Autodesk Fusion 360 part; units mm, degrees
sketch "Sketch1" plane through (0, 0, 0) normal (0, 1, 0) x (1, 0, 0)
  line L0 (-25, 0) -> (15, 0)
  line L1 (15, 0) -> (15, -10)
  line L2 (15, -10) -> (-25, -10)
  line L3 (-25, -10) -> (-25, 0)
  dimension "d1" = 40
  dimension "d2" = 10
extrude "Extrude1" add sketch "Sketch1" along normal blind 16
sketch "Sketch2" plane through (0, 16, 0) normal (0, 1, 0) x (-1, 0, 0)
  line L0 (25, 10) -> (-15, 10)
  line L1 (-15, 10) -> (-15, 0)
  line L2 (-15, 0) -> (25, 0)
  line L3 (25, 0) -> (25, 10)
  line L4 (-15, 10) -> (-3, 10)
  line L5 (-3, 10) -> (-3, 9)
  line L6 (-3, 9) -> (6.5, 9)
  line L7 (6.5, 9) -> (6.5, 1)
  line L8 (6.5, 1) -> (-3, 1)
  line L9 (-3, 1) -> (-3, 9)
  dimension "d5" = 12
  dimension "d6" = 9.5
  dimension "d7" = 8
extrude "Extrude2" cut sketch "Sketch2" against normal blind 50 contours L6 L7 L8 L9
sketch "Sketch3" plane through (0, 0, 10) normal (0, 0, 1) x (1, 0, 0)
  line L0 (-25, 0) -> (15, 0)
  line L1 (15, 0) -> (15, 16)
  line L2 (15, 16) -> (-25, 16)
  line L3 (-25, 16) -> (-25, 0)
  line L4 (15, 16) -> (3, 16)
  line L5 (3, 16) -> (3, 12.75)
  line L6 (3, 12.75) -> (-6.5, 12.75)
  line L7 (-6.5, 12.75) -> (-6.5, 16)
  line L8 (-6.5, 16) -> (3, 16)
  line L9 (3, 16) -> (3, 12.75)
  line L10 (-6.5, 12.75) -> (3, 12.75)
  line L11 (3, 12.75) -> (3, -1)
  line L12 (3, -1) -> (-6.5, -1)
  line L13 (-6.5, -1) -> (-6.5, 12.75)
  dimension "d10" = 12
  dimension "d11" = 3.25
  dimension "d12" = 9.5
extrude "Extrude3" cut sketch "Sketch3" against normal blind 50 contours L0 L6 L10 L11 L13
sketch "Sketch4" plane through (0, 0, 10) normal (0, 0, 1) x (1, 0, 0)
  line L0 (-6.5, 0) -> (-6.5, 12.75)
  line L1 (-6.5, 12.75) -> (3, 12.75)
  line L2 (3, 12.75) -> (3, 0)
  line L3 (3, 0) -> (15, 0)
  line L4 (15, 0) -> (15, 16)
  line L5 (15, 16) -> (-25, 16)
  line L6 (-25, 16) -> (-25, 0)
  line L7 (-25, 0) -> (-6.5, 0)
  line L8 (-25, 12.75) -> (-20, 12.75)
  line L9 (-20, 12.75) -> (-20, -3.5611)
  line L10 (-20, -3.5611) -> (-25, -3.5611)
  line L11 (-25, -3.5611) -> (-25, 12.75)
  line L12 (15, 12.75) -> (10, 12.75)
  line L13 (10, 12.75) -> (10, -3.5611)
  line L14 (10, -3.5611) -> (15, -3.5611)
  line L15 (15, -3.5611) -> (15, 12.75)
  dimension "d15" = 5
  dimension "d16" = 5
extrude "Extrude4" cut sketch "Sketch4" against normal blind 50 contours L7 L9 L10 L11 | L6 L7 L8 L9 L11 | L3 L4 L12 L13 L15 | L3 L13 L14 L15
sketch "Sketch5" plane through (0, 16, 0) normal (0, 1, 0) x (-1, 0, 0)
  line L0 (6.5, 9) -> (6.5, 1)
  line L1 (6.5, 1) -> (-3, 1)
  line L2 (-3, 1) -> (-3, 9)
  line L3 (-3, 9) -> (6.5, 9)
  line L4 (25, 10) -> (-15, 10)
  line L5 (-15, 10) -> (-15, 0)
  line L6 (-15, 0) -> (25, 0)
  line L7 (25, 0) -> (25, 10)
  line L8 (-3, 1) -> (-5.5, 1)
  line L9 (-5.5, 1) -> (-5.5, 8.9913)
  line L10 (-5.5, 8.9913) -> (-3, 8.9913)
  line L11 (-3, 8.9913) -> (-3, 1)
  dimension "d19" = 2.5
extrude "Extrude5" cut sketch "Sketch5" against normal blind 13.5 contours L2 L8 L9 L10 L11
sketch "Sketch6" plane through (0, 0, 10) normal (0, 0, 1) x (1, 0, 0)
  line L0 (-25, 12.75) -> (-20, 12.75)
  line L1 (-20, 12.75) -> (-20, 0)
  line L2 (-20, 0) -> (-6.5, 0)
  line L3 (-6.5, 0) -> (-6.5, 12.75)
  line L4 (-6.5, 12.75) -> (3, 12.75)
  line L5 (3, 12.75) -> (3, 0)
  line L6 (3, 0) -> (10, 0)
  line L7 (10, 0) -> (10, 12.75)
  line L8 (10, 12.75) -> (15, 12.75)
  line L9 (15, 12.75) -> (15, 16)
  line L10 (15, 16) -> (-25, 16)
  line L11 (-25, 16) -> (-25, 12.75)
  line L12 (-6.5, 0) -> (-6.5, 0.3)
  line L13 (-6.5, 0) -> (-9.5, 0)
  line L14 (-9.5, 0) -> (-6.5, 0.3)
  dimension "d22" = 0.3
  dimension "d23" = 3
extrude "Extrude6" cut sketch "Sketch6" against normal blind 50 contours L2 L3 L12 L13 L14
sketch "Sketch7" plane through (3, 0, 0) normal (-1, 0, 0) x (0, 0, 1)
  line L0 (8.9913, 16) -> (8.9913, 2.5)
  line L1 (8.9913, 2.5) -> (1, 2.5)
  line L2 (1, 2.5) -> (1, 12.75)
  line L3 (1, 12.75) -> (0, 12.75)
  line L4 (0, 12.75) -> (0, 0)
  line L5 (0, 0) -> (10, 0)
  line L6 (10, 0) -> (10, 12.75)
  line L7 (10, 12.75) -> (9, 12.75)
  line L8 (9, 12.75) -> (9, 16)
  line L9 (9, 16) -> (8.9913, 16)
  line L10 (10, 0) -> (8.2, 0)
  line L11 (8.2, 0) -> (8.85, 0)
  line L12 (8.85, 0) -> (5.6472, 1.5221)
  line L13 (8.85, 0) -> (12.3961, 0) construction
  line L14 (5.6472, 1.5221) -> (4.9972, 1.5221)
  line L15 (4.9972, 1.5221) -> (8.2, 0)
  line L16 (0, 0) -> (1.8, 0)
  line L17 (1.8, 0) -> (1.15, 0)
  line L18 (1.15, 0) -> (4.3528, 1.5221)
  line L19 (4.3528, 1.5221) -> (5.0028, 1.5221)
  line L20 (4.9972, 1.5221) -> (1.8, 0)
  line L21 (4.3528, 1.5221) -> (5.6, 1.5221)
  line L22 (5.6, 1.5221) -> (5.6, 1.7721)
  line L23 (5.6, 1.7721) -> (4.3528, 1.7721)
  line L24 (4.3528, 1.7721) -> (4.3528, 1.5221)
  dimension "d26" = 1.8
  dimension "d27" = 0.65
  dimension "d28" = 154.581
  dimension "d29" = 3.5461
  dimension "d30" = 0.65
  dimension "d31" = 1.8
  dimension "d32" = 0.65
  dimension "d33" = 3.5461
  dimension "d34" = 25.419
  dimension "d35" = 0.65
  dimension "d36" = 0.25
extrude "Extrude7" cut sketch "Sketch7" along normal blind 20 and the other way blind 5 contours L5 L10 L11 L12 L14 L15 L19 L21 | L5 L16 L17 L18 L19 L20 L21 | L14 L19 L21 L22 L23 L24
sketch "Sketch8" plane through (3, 0, 0) normal (-1, 0, 0) x (0, 0, 1)
  line L0 (5.6472, 1.5221) -> (8.85, 0)
  line L1 (8.85, 0) -> (10, 0)
  line L2 (10, 0) -> (10, 12.75)
  line L3 (10, 12.75) -> (9, 12.75)
  line L4 (9, 12.75) -> (9, 16)
  line L5 (9, 16) -> (8.9913, 16)
  line L6 (8.9913, 16) -> (8.9913, 2.5)
  line L7 (8.9913, 2.5) -> (1, 2.5)
  line L8 (1, 2.5) -> (1, 12.75)
  line L9 (1, 12.75) -> (0, 12.75)
  line L10 (0, 12.75) -> (0, 0)
  line L11 (0, 0) -> (1.15, 0)
  line L12 (1.15, 0) -> (4.3528, 1.5221)
  line L13 (4.3528, 1.5221) -> (4.3528, 1.7721)
  line L14 (4.3528, 1.7721) -> (5.6, 1.7721)
  line L15 (5.6, 1.7721) -> (5.6, 1.5221)
  line L16 (5.6, 1.5221) -> (5.6472, 1.5221)
  line L17 (5.6, 1.5221) -> (8.85, 0)
  line L18 (8.85, 0) -> (8.95, 0)
  line L19 (5.6, 1.5221) -> (5.7, 1.5221)
  line L20 (5.7, 1.5221) -> (8.95, 0)
  line L21 (1.15, 0) -> (1.05, 0)
  line L22 (1.15, 0) -> (4.3528, 1.5221)
  line L23 (4.3528, 1.5221) -> (4.2528, 1.5221)
  line L24 (4.2528, 1.5221) -> (1.05, 0)
  line L25 (4.1564, 1.7721) -> (5.7264, 1.7721)
  line L26 (5.7264, 1.7721) -> (5.7264, 1.5221)
  line L27 (5.7264, 1.5221) -> (4.1564, 1.5221)
  line L28 (4.1564, 1.5221) -> (4.1564, 1.7721)
  dimension "d41" = 0.1
  dimension "d42" = 0.1
  dimension "d43" = 0.1
  dimension "d44" = 0.25
extrude "Extrude8" cut sketch "Sketch8" along normal blind 20 and the other way blind 5 contours L0 L16 L17 L19 L27 | L15 L16 L19 L25 L26 L27 | L13 L14 L15 L25 L27 | L13 L23 L25 L27 L28 | L11 L12 L21 L22 L23 L24 L27
sketch "Sketch9" plane through (3, 0, 0) normal (-1, 0, 0) x (0, 0, 1)
  line L0 (1.05, 0) -> (4.2528, 1.5221)
  line L1 (4.2528, 1.5221) -> (4.1564, 1.5221)
  line L2 (4.1564, 1.5221) -> (4.1564, 1.7721)
  line L3 (4.1564, 1.7721) -> (5.7264, 1.7721)
  line L4 (5.7264, 1.7721) -> (5.7264, 1.5221)
  line L5 (5.7264, 1.5221) -> (5.6472, 1.5221)
  line L6 (5.6472, 1.5221) -> (8.85, 0)
  line L7 (8.85, 0) -> (10, 0)
  line L8 (10, 0) -> (10, 12.75)
  line L9 (10, 12.75) -> (9, 12.75)
  line L10 (9, 12.75) -> (9, 16)
  line L11 (9, 16) -> (8.9913, 16)
  line L12 (8.9913, 16) -> (8.9913, 2.5)
  line L13 (8.9913, 2.5) -> (1, 2.5)
  line L14 (1, 2.5) -> (1, 12.75)
  line L15 (1, 12.75) -> (0, 12.75)
  line L16 (0, 12.75) -> (0, 0)
  line L17 (0, 0) -> (1.05, 0)
  line L18 (1.05, 0) -> (0.8, 0)
  line L19 (4.2528, 1.5221) -> (4.0028, 1.5221)
  line L20 (4.0028, 1.5221) -> (0.8, 0)
  line L21 (1.05, 0) -> (4.2528, 1.5221)
  line L22 (8.85, 0) -> (9.1, 0)
  line L23 (5.6472, 1.5221) -> (5.8972, 1.5221)
  line L24 (5.8972, 1.5221) -> (9.1, 0)
  line L25 (8.85, 0) -> (5.6472, 1.5221)
  line L26 (4.0028, 1.5221) -> (5.8972, 1.5221)
  line L27 (5.8972, 1.5221) -> (5.8972, 1.8221)
  line L28 (5.8972, 1.8221) -> (4.0028, 1.8221)
  line L29 (4.0028, 1.8221) -> (4.0028, 1.5221)
  dimension "d49" = 0.25
  dimension "d50" = 0.25
  dimension "d51" = 0.25
  dimension "d52" = 0.3
extrude "Extrude9" cut sketch "Sketch9" along normal blind 20 and the other way blind 5 contours L0 L1 L17 L18 L19 L20 L21 L26 | L1 L2 L3 L4 L5 L19 L23 L26 | L2 L3 L4 L19 L23 L26 L27 L28 L29 | L5 L6 L7 L22 L23 L24 L25 L26
sketch "Sketch10" plane through (3, 0, 0) normal (-1, 0, 0) x (0, 0, 1)
  line L0 (0.8, 0) -> (4.0028, 1.5221)
  line L1 (4.0028, 1.5221) -> (4.0028, 1.8221)
  line L2 (4.0028, 1.8221) -> (5.8972, 1.8221)
  line L3 (5.8972, 1.8221) -> (5.8972, 1.5221)
  line L4 (5.8972, 1.5221) -> (9.1, 0)
  line L5 (9.1, 0) -> (10, 0)
  line L6 (10, 0) -> (10, 12.75)
  line L7 (10, 12.75) -> (9, 12.75)
  line L8 (9, 12.75) -> (9, 16)
  line L9 (9, 16) -> (8.9913, 16)
  line L10 (8.9913, 16) -> (8.9913, 2.5)
  line L11 (8.9913, 2.5) -> (1, 2.5)
  line L12 (1, 2.5) -> (1, 12.75)
  line L13 (1, 12.75) -> (0, 12.75)
  line L14 (0, 12.75) -> (0, 0)
  line L15 (0, 0) -> (0.8, 0)
  line L16 (1.8, 0) -> (5, 1.4019)
  line L17 (1.8, 0) -> (5.2936, 0) construction
  line L18 (8.2, 0) -> (5, 1.4019)
  line L19 (8.2, 0) -> (11.6936, 0) construction
  line L20 (8.2, 0) -> (8.2, 0.2)
  line L21 (8.2, 0.2) -> (4.9, 1.7)
  line L22 (4.9, 1.7) -> (1.4, 0)
  line L23 (1.4, 0) -> (1.8, 0)
  line L24 (4.0028, 1.8221) -> (4.0028, 2)
  line L25 (4.0028, 2) -> (5.9, 2)
  line L26 (5.8972, 1.8221) -> (5.9, 2)
  line L27 (5.8972, 1.8221) -> (4.0028, 1.8221)
  dimension "d57" = 23.658
  dimension "d58" = 3.4936
  dimension "d59" = 156.342
  dimension "d60" = 3.4936
sketch "Sketch11" plane through (3, 0, 0) normal (-1, 0, 0) x (0, 0, 1)
sketch "Sketch12" plane through (3, 0, 0) normal (-1, 0, 0) x (0, 0, 1)
  line L0 (8.2, 0) -> (4.9972, 1.5221)
  line L1 (4.9972, 1.5221) -> (1.8, 0)
  line L2 (1.8, 0) -> (8.2, 0)
  line L3 (1.8, 0) -> (4.9972, 1.5221)
  line L4 (4.9972, 1.5221) -> (8.2, 0)
  line L5 (8.2, 0) -> (5, 1.4)
  line L6 (5, 1.4) -> (1.8, 0)
extrude "Extrude10" cut sketch "Sketch10" sketch "Sketch12" along normal blind 20 and the other way blind 5 contours L2 L24 L25 L26 L27 of sketch 2 contours L0 L1 L3 L4 L5 L6
Source: CAD feature listing. Evaluate the final solid. Frame: model axes, mm. A direction names the side the tool comes from. Coordinates: 2 decimals unless noted, no trailing zeros. Write each loop counter-clockwise with the first axis right and the second up, starting at its lowest first coordinate (ties: lowest second). Pieces come first, ordered by that corner, then holes. Notation, with made-up numbers: M 54,44 L 71,44 A5 ccw 71,50 Z; hole C 40.25,59.5 d8. An arc over 180 degrees is marked long. Answer as a JSON object with one key per item and string values.
1. Cut plane C-C on z = 6.5. Output: boundary loops of the cut face in (x, y).
Evaluation:
{"outline": "M -25,12.75 L -20,12.75 L -20,0 L -9.5,0 L -6.5,0.3 L -6.5,0.74 L -17,0.74 L -17,1.24 L -6.5,1.24 L -6.5,16 L -25,16 Z; M 3,0 L 10,0 L 10,12.75 L 15,12.75 L 15,16 L 5.5,16 L 5.5,2.5 L 3,2.5 L 3,1.24 L 8,1.24 L 8,0.74 L 3,0.74 Z"}
2. Cut plane A-A on y = 5.5. Output: boundary loops of the cut face in (x, z), plus the area to 3 significant figures.
Evaluation:
{"outline": "M -20,0 L -6.5,0 L -6.5,10 L -20,10 Z; M 3,0 L 10,0 L 10,10 L 3,10 L 3,8.99 L 5.5,8.99 L 5.5,1 L 3,1 Z", "area": "185 mm^2"}
3. Ray query, L1, parallel to X at y = 2.75, z = 0.75; L2, parallel to Y at x = -15.5, z = 2.5; L3, parallel to Z at x = 6, y = 1. Return the intervals inside material, ascending.
Evaluation:
{"L1": "-20 to -6.5, 3 to 10", "L2": "0 to 0.31, 0.81 to 16", "L3": "0 to 2.9, 4.09 to 5.91, 7 to 10"}
4. Contact query for flat-ended pins moving along their axis: P1, Ø1.5, axis at x = 11.5, z = 7, coming from the -Y side; P2, Ø1, axis at y = 1, z = 5.5, coming from the +X side; P3, Ø6, axis at y = 3, z = 6.5, coming from the -X side. Output: stop coordinate, or through.
Evaluation:
{"P1": "y = 12.75", "P2": "x = 10", "P3": "x = -20"}
5. Access query for faces 4 (the flat face through (5.5, 0.7, 6.6)), 5 (the flat face through (3, 1, 5)), 6 (the flat face through (13, 12.75, 5)), 7 (the flat face through (-8.02, 0.15, 9.42)), 8 (the flat face through (5.5, 9, 5)). Directions: +Z, -Z, +X, -X, +Y, -Y. A direction counts if a zero-diameter tool reaches every point of the face in a straight line with its end or side. Return the directions, or none.
Evaluation:
{"face 4": "none", "face 5": "+Z, -Z, +Y, -Y", "face 6": "+Z, -Z, +X, -Y", "face 7": "+Z, -Z, -Y", "face 8": "+Y"}
6. Draft query along Z for faces 1 (the flat face through (10, 6, 5)), 2 (the flat face through (6, 2, 5)), 3 (the flat face through (4, 9, 8.991)). Return one class per face: released by +Z, released by -Z, zero draft, split by the parting line, or undercut.
Evaluation:
{"face 1": "zero draft", "face 2": "undercut", "face 3": "undercut"}
7. Cut plane B-B on x = -16.5. Output: boundary loops of the cut face in (y, z), plus the area to 3 significant figures.
Evaluation:
{"outline": "M 0,0 L 16,0 L 16,10 L 0,10 L 0,9.1 L 1.52,5.9 L 1.82,5.9 L 2,5.9 L 2,4 L 1.52,4 L 0,0.8 Z; M 0,1.8 L 1.4,5 L 0,8.2 Z", "area": "156 mm^2"}
